Can you work these out from the model? Positions are in its coordinate system, mm. Face numbers are marked on the shaded views. Coordinates: 2 decimals unless noted, no trailing zeros. Order: outer loops, then holes, each group sorted by start corner. A loop starts at its lowest first (then second) coordinate and runs counter-clockwise, first axis right, second up.
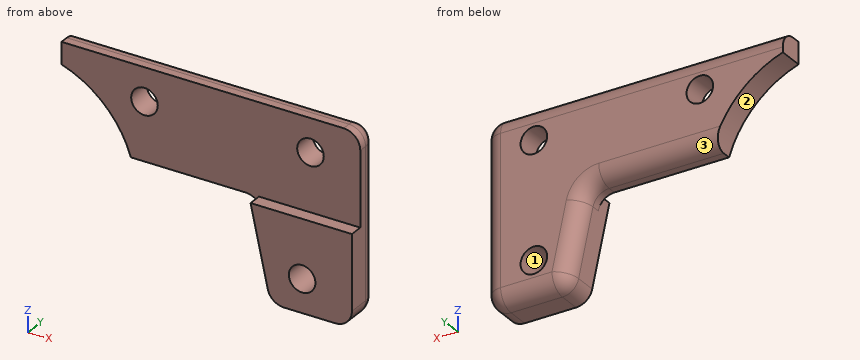
Autodesk Inventor part; units mm, degrees
ref_plane "YZ Plane" through (0, 0, 0) normal (1, 0, 0) x (0, 1, 0)
ref_plane "XZ Plane" through (0, 0, 0) normal (0, 1, 0) x (-1, 0, 0)
ref_plane "XY Plane" through (0, 0, 0) normal (0, 0, 1) x (1, 0, 0)
sketch "スケッチ1" plane through (0, 0, 0) normal (0, 1, 0) x (-1, 0, 0)
  line L0 (20, 0) -> (0, 0)
  line L1 (0, 0) -> (0, -27)
  line L2 (0, -27) -> (20, -27)
  line L3 (20, -27) -> (20, 0)
  circle A0 centre (20, -13.5) radius 13.5
  circle A1 centre (20, -13.5) radius 14
  circle A2 centre (20, -13.5) radius 2
  line L4 (20, -11.5) -> (-0.0059, -11.5)
  line L5 (0, -27) -> (20, -27)
  line L6 (20, -27) -> (20, -17)
  line L7 (20, -17) -> (0, -17)
  line L8 (0, -17) -> (0, -27)
  line L9 (20, -11.5) -> (0, -11.5)
  line L10 (0, -11.5) -> (0, -6)
  line L11 (0, -6) -> (20, -6)
  line L12 (20, -6) -> (20, -11.5)
  circle A3 centre (20, -13.5) radius 6.5
  line L13 (20, -10.5) -> (-0.0015, -10.5)
  line L14 (6.3252, -10.5) -> (2.7054, -27)
  point P0 (16.2919, 0)
  point P1 (16.2919, -27)
  point P2 (0, -11.5)
  point P3 (6.1436, -11.5)
  point P4 (0, -17)
  point P5 (6.4446, -17)
  point P6 (8.1784, -6)
  point P7 (13.8153, -11.5)
  point P8 (20, -7)
  point P9 (14.5228, -17)
  point P10 (20, -20)
  point P11 (6.1058, -11.5)
  point P12 (4.8992, -17)
  dimension "d1" = 28
  dimension "d2" = 4
  dimension "d0" = 27
  dimension "d7" = 20
  dimension "d8" = 10
  dimension "d9" = 5.5
  dimension "d21" = 13
  dimension "d22" = 1
extrude "押し出し1" add sketch "スケッチ1" along normal blind 2.3 contours L3 A3 L13 A0 L11 | A0 L13 A1 L11 | A1 L13 L1 L11 | L13 A3 L4 A0 | A0 L4 A1 L13 | L14 L4 L1 L13 | A1 L4 L14 | L14 L7 L1 L4
extrude "押し出し2" cut sketch "スケッチ1" along normal blind 0.8 contours A1 L11 L1 L0 | L3 A3 L13 A0 L11 | A0 L13 A1 L11 | A1 L13 L1 L11 | L13 A3 L4 A0 | A0 L4 A1 L13 | L14 L4 L1 L13 | A1 L4 L14
sketch "スケッチ2" plane through (0, 2.3, 0) normal (0, 1, 0) x (1, 0, 0)
  circle A0 centre (-3, 15) radius 0.8
  line L0 (-20, 6) -> (0, 6)
  line L1 (0, 0) -> (0, 17)
  circle A1 centre (-3, 8) radius 0.8
  line L2 (0, 17) -> (-4.8992, 17)
  circle A2 centre (-13, 8) radius 0.8
  circle A3 centre (-13, 8) radius 0.8
  circle A4 centre (-3, 8) radius 0.8
  line L3 (-18, 0) -> (-18, 7.3153)
  line L4 (-18, 0) -> (0.4606, 0)
  line L5 (0.4606, 0.5589) -> (0.4606, 0)
  arc A5 (0.4606, 5.4411) -> (0.4606, 0.5589) centre (1, 3) ccw
  line L6 (0.4606, 10.5) -> (0.4606, 5.4411)
  line L7 (0.4606, 10.5) -> (-14.2337, 10.5)
  arc A6 (-18, 7.3153) -> (-14.2337, 10.5) centre (-20, 13.5) ccw
  arc A7 (-20, 7) -> (-13.8153, 11.5) centre (-20, 13.5) ccw
  line L8 (-20, 7) -> (-20, 6)
  line L9 (-20, 6) -> (0, 6)
  line L10 (0, 6) -> (0, 17)
  line L11 (0, 17) -> (-4.8992, 17)
  line L12 (-4.8992, 17) -> (-6.1058, 11.5)
  line L13 (-6.1058, 11.5) -> (-13.8153, 11.5)
  point P0 (-8.1784, 6)
  point P1 (-6.4446, 17)
  point P2 (-5.3497, 17)
  point P3 (0, 27)
  point P4 (-14.5228, 17)
  point P5 (-20, 17)
  point P6 (-18, 6)
  dimension "d11" = 1.6
  dimension "d14" = 1.6
  dimension "d15" = 2
  dimension "d16" = 3
  dimension "d17" = 2
  dimension "d23" = 1.6
  dimension "d24" = 10
extrude "押し出し3" cut sketch "スケッチ2" against normal through all contours A0 | L8 A7 L3 L0 | A1 | A2
fillet "フィレット1" radius 1 9 edges at (0, 1.55, -6) (0, 1.15, -17) (-9, 2.3, -6) (0, 2.3, -11.5) (-2.4496, 2.3, -17) (-9.9606, 2.3, -11.5) (-5.5025, 2.3, -14.25) (-4.8992, 1.15, -17) (-6.1058, 1.55, -11.5)
properties part number "leg_springjoint_cover_under_left"
1. Imagine slicing it at A-A on x = -3. Please give me the cut outline in (y, z), then the cut area to 3 significant figures.
Completed:
outline: (0, -17) - (1.3, -17) arc R1 ccw to (2.3, -16) - (2.3, -15.8) - (0, -15.8) - close; (0, -14.2) - (2.3, -14.2) - (2.3, -8.8) - (0.8, -8.8) - (0.8, -11.5) - (0, -11.5) - close; (0.8, -7.2) - (2.3, -7.2) - (2.3, -7) arc R1 ccw to (1.3, -6) - (0.8, -6) - close
area: 14.4 mm2
2. Please list where these lines run through material, in increasing order: probe 1 along Z at (x, y) = (-3, 0.6); probe 2 along X at (y, z) = (1.5, -8); probe 3 along Z at (x, y) = (-3, 1.8).
Completed:
probe 1: z = -17 to -15.8, -14.2 to -11.5
probe 2: x = -16.54 to -13.8, -12.2 to -3.8, -2.2 to -0.02
probe 3: z = -16.87 to -15.8, -14.2 to -8.8, -7.2 to -6.13
3. Imagine slicing it at B-B on z = -8. Please give me the cut outline in (x, y).
Completed:
outline: (-16.54, 0.8) - (-13.8, 0.8) - (-13.8, 2.3) - (-16.54, 2.3) - close; (-12.2, 0.8) - (-3.8, 0.8) - (-3.8, 2.3) - (-12.2, 2.3) - close; (-2.2, 0.8) - (0, 0.8) - (0, 1.3) arc R1 ccw to (-1, 2.3) - (-2.2, 2.3) - close
4. I'm going to push flat-ended pins straight in: pin 1 (1 mm diameter, centred on y = 1.5, z = -11.5, fed in from +X); pin 2 (3 mm diameter, centred on x = -13.5, z = -8.5, fed in from -Y); pin 3 (1.4 mm diameter, centred on x = -3, z = -8, fed in from -Y); pin 4 (0.6 mm diameter, centred on x = -9.5, y = 1, fed in from -Z). Where does each tip first touch, or does it pass through?
Completed:
pin 1: stops at x = 0
pin 2: stops at y = 0.8
pin 3: passes through
pin 4: stops at z = -11.5
5. Imagine slicing it at D-D on y = 1.6. Please give me the cut outline in (x, z).
Completed:
outline: (-18, -7.32) arc R6.5 cw to (-13.83, -11.45) - (-6.91, -11.45) arc R1.05 cw to (-5.89, -12.28) - (-5.03, -16.2) arc R0.95 ccw to (-4.09, -16.95) - (-1, -16.95) arc R0.95 ccw to (-0.05, -16) - (-0.05, -7) arc R0.95 ccw to (-1, -6.05) - (-18, -6.05) - close; hole circle Ø1.6 at (-13, -8); hole circle Ø1.6 at (-3, -15); hole circle Ø1.6 at (-3, -8)
6. Imagine slicing it at C-C on x = -13. Please give me the cut outline in (y, z), then the cut area to 3 significant figures.
Completed:
outline: (0.8, -11.5) - (1.3, -11.5) arc R1 ccw to (2.3, -10.5) - (2.3, -8.8) - (0.8, -8.8) - close; (0.8, -7.2) - (2.3, -7.2) - (2.3, -7) arc R1 ccw to (1.3, -6) - (0.8, -6) - close
area: 5.42 mm2
7. Thinking about a two-plate mould opening in X: for the marked faces 1, 2 and 3, which applies, pulls with the +X half, pulls with the -X half, needs draft (parallel to the pull), parting line crosses it, or undercut?
Completed:
face 1: undercut
face 2: pulls with the -X half
face 3: needs draft
